Verification items for the finished model (mm, model axes). A direction names the side the tool comes from. Round coordinates to 2 decimals unless told otherwise and drop trailing zeros. Write each loop counter-clockwise with the first axis right and the second up, starting at its lowest first coordinate (ties: lowest second). Pieces come first, ordered by that corner, then holes.
from build123d import *

# Parameters (mm, degrees)
F0_R     = 25.4
F1_DEPTH = 50.8
F2_R     = 3.175
F3_DEPTH = 50.8
F4_R     = 10.183326
F5_DEPTH = 25.4
F6_W     = 24.701291
F6_H     = 17.974584
F7_DEPTH = 50.8


with BuildPart() as f1:
    # F0 (on Front) → F1 (new body)
    with BuildSketch(Plane.XZ):
        Circle(F0_R)
    extrude(amount=F1_DEPTH)

    # F2 (on face) → F3 (cut, through all)
    with BuildSketch(Plane.XZ.offset(50.8)):
        with Locations((0, 12.7)):
            Circle(F2_R)
        with Locations((12.7, 0)):
            Circle(F2_R)
        with Locations((0, -12.7)):
            Circle(F2_R)
        with Locations((-12.7, 0)):
            Circle(F2_R)
    extrude(amount=-F3_DEPTH, mode=Mode.SUBTRACT)

    # F4 (on face) → F5 (cut)
    with BuildSketch(Plane.XZ.offset(50.8)):
        with Locations((0, -2.647925)):
            Circle(F4_R)
    extrude(amount=-F5_DEPTH, mode=Mode.SUBTRACT)

    # F6 (on face) → F7 (cut)
    with BuildSketch(Plane.XZ.offset(50.8)):
        with Locations((2.291639, 3.951871)):
            Rectangle(F6_W, F6_H)
    extrude(amount=-F7_DEPTH, mode=Mode.SUBTRACT)


solid = f1.part
Q1. Sectioned sample at A-A (y = -8). Enter the section's corners in (x, z) (3 decimals).
Recorded:
outline: circle Ø50.8 at (0, 0); hole (-10.059, -5.035) - (14.642, -5.035) - (14.642, -2.512) arc R3.175 ccw to (14.642, 2.512) - (14.642, 12.939) - (3.166, 12.939) arc R3.175 ccw to (-3.166, 12.939) - (-10.059, 12.939) - (-10.059, 1.762) arc R3.175 ccw (long way) to (-10.059, -1.762) - close; hole circle Ø6.35 at (0, -12.7)
Q2. Sectioned sample at C-C (z = 0). Enter the section's corners in (x, y) (3 decimals), plus the area to 3 significant figures.
Recorded:
outline: (-25.4, -50.8) - (-15.875, -50.8) - (-15.875, 0) - (-25.4, 0) - close; (15.875, -50.8) - (25.4, -50.8) - (25.4, 0) - (15.875, 0) - close
area: 968 mm2
Q3. Sectioned sample at D-D (x = 8). Enter the section's corners in (y, z).
Recorded:
outline: (-50.8, -24.11) - (0, -24.11) - (0, -5.04) - (-25.4, -5.04) - (-25.4, -8.95) - (-50.8, -8.95) - close; (-50.8, 12.94) - (0, 12.94) - (0, 24.11) - (-50.8, 24.11) - close
Q4. Sectioned sample at B-B (x = 0). Enter the section's corners in (y, z) (3 decimals).
Recorded:
outline: (-50.8, -25.4) - (0, -25.4) - (0, -15.875) - (-50.8, -15.875) - close; (-50.8, 15.875) - (0, 15.875) - (0, 25.4) - (-50.8, 25.4) - close; (-25.4, -9.525) - (0, -9.525) - (0, -5.035) - (-25.4, -5.035) - close
Q5. Material ranges on line 1 along Z through (x, y) = (2, -6.5); line 2 along Z through (x, y) = (0, -36) (3 decimals); line 3 along X through (y, z) = (-47.5, -14.5), recorded low to high.
Recorded:
line 1: z = -25.32 to -15.17, -10.23 to -5.04, 15.17 to 25.32
line 2: z = -25.4 to -15.875, 15.875 to 25.4
line 3: x = -20.85 to -2.62, 2.62 to 20.85
Q6. Tool access check on faces 4 (the flat face through (-0.4, 0, -5.3)), 5 (the flat face through (14.642, -26, -4)), 6 (the cylindrical face through (-10.175, -38.278, -3.053)). Record the directions out of +Z, -Z, +X, -X, +Y, -Y that give a thin tool (end or side, any length) a straight path to the whole face; none if there is none.
Recorded:
face 4: +Z, -Z, +X, -X, +Y
face 5: +Y, -Y
face 6: -Y
Q7. Release check for a two-part mould opening along Z. For faces 1 (the flat face through (-10.059, -26, 7)), 2 (the flat face through (10.9, -50.8, -5.3)), 3 (the cylindrical face through (-5.506, -25.044, -24.796)) record: released by +Z, released by -Z, zero draft, split by the parting line, or undercut.
Recorded:
face 1: undercut
face 2: zero draft
face 3: split by the parting line
Q8. Depth check by flat-ended pin: P1, Ø9, axis at x = 7, y = -19, coming from the -Z side; P2, Ø3.5, axis at y = -13, z = 6.5, coming from the +X side; P3, Ø4, axis at x = 0.5, z = -6, coming from the -Y side; P4, Ø4, axis at x = 0, z = -12.7, coming from the +Y side. Enter the tip coordinate at first touch or a pass-through.
Recorded:
P1: stops at z = -25.28
P2: stops at x = 24.95
P3: stops at y = -25.4
P4: passes through
